```python
from build123d import *

# Parameters (mm, degrees)
F0_W     = 101.6
F0_H     = 114.3
F1_DEPTH = 19.05
F3_D     = 6.7564


# Not quite as in the source:
# - a feature names something its author has since deleted; it is built from what else it names


with BuildPart() as f1:
    # F0 (on Top) → F1 (new body)
    with BuildSketch(Plane.XY):
        Rectangle(F0_W, F0_H)
    extrude(amount=F1_DEPTH)

    # F3 (through all)
    with Locations(Plane.XY.offset(19.05)):
        with Locations((-30.48, -47.625), (-10.16, -47.625), (10.16, -47.625), (30.48, -47.625), (-19.05, 47.625), (-25.4, 11.0744), (-25.4, -22.225), (-8.4666666667, -22.225), (-8.4666666667, 11.0744), (8.4666666667, 11.0744), (8.4666666667, -22.225), (25.4, -22.225), (25.4, 11.0744), (19.05, 47.625), (-19.05, 28.575), (19.05, 28.575)):
            Hole(F3_D / 2)


solid = f1.part
```
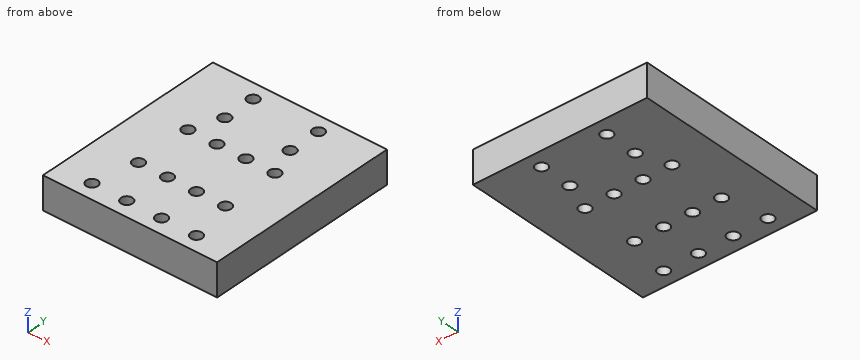
Verification items for the finished model (mm, model axes). Give positions to 0.01 mm unless a question says otherwise; leave off trailing zeros. Loops run counter-clockwise (first coordinate to the right, second up) from the corner with the lowest first, then second, coordinate; pieces in that order, holes last.
1. Section check A-A, the plane x = 30.48. Enter the section's corners in (y, z), then the cut area to 3 significant figures.
2. Section check B-B, the plane x = -19.05. Enter the section's corners in (y, z), then the cut area to 3 significant figures.
3. Section check C-C, the plane y = -46. Enter the section's corners in (x, z), then the cut area to 3 significant figures.
4. Section check D-D, the plane z = 4.75. Count the separate pieces of the cut face and the enclosed holes in it, then the cut area to 3 significant figures.
5. Thickness scan on line 1 (Y direction, x = 21, z = 7); line 2 (X direction, y = -45, z = 4.5); line 3 (X direction, y = 9, z = 4). Record the ranges inside material, lowest first.
6. Go/stop test with a flat-tipped pin: pin 1 Ø8 at (x, y) = (25.4, -22.225) entering from -Z. Record where the tip stops, or that it passes through.
Geometry says:
1. outline: (-57.15, 0) - (-51, 0) - (-51, 19.05) - (-57.15, 19.05) - close; (-44.25, 0) - (57.15, 0) - (57.15, 19.05) - (-44.25, 19.05) - close
1. area: 2,050 mm2
2. outline: (-57.15, 0) - (25.2, 0) - (25.2, 19.05) - (-57.15, 19.05) - close; (31.95, 0) - (44.25, 0) - (44.25, 19.05) - (31.95, 19.05) - close; (51, 0) - (57.15, 0) - (57.15, 19.05) - (51, 19.05) - close
2. area: 1,920 mm2
3. outline: (-50.8, 0) - (-33.44, 0) - (-33.44, 19.05) - (-50.8, 19.05) - close; (-27.52, 0) - (-13.12, 0) - (-13.12, 19.05) - (-27.52, 19.05) - close; (-7.2, 0) - (7.2, 0) - (7.2, 19.05) - (-7.2, 19.05) - close; (13.12, 0) - (27.52, 0) - (27.52, 19.05) - (13.12, 19.05) - close; (33.44, 0) - (50.8, 0) - (50.8, 19.05) - (33.44, 19.05) - close
3. area: 1,480 mm2
4. separate pieces: 1
4. enclosed holes: 16
4. area: 11,000 mm2
5. line 1: y = -57.15 to 25.82, 31.33 to 44.87, 50.38 to 57.15
5. line 2: x = -50.8 to -32.61, -28.35 to -12.29, -8.03 to 8.03, 12.29 to 28.35, 32.61 to 50.8
5. line 3: x = -50.8 to -28.07, -22.73 to -11.13, -5.8 to 5.8, 11.13 to 22.73, 28.07 to 50.8
6. pin 1: stops at z = 0
